```python
from build123d import *

# Parameters (mm, degrees)
ESQUISSE1_R                  = 30.9
ESQUISSE1_R_2                = 12.5
BOSS_EXTRU_1_DEPTH           = 0.6
ESQUISSE2_R                  = 2.1
ENL_V_MAT_EXTRU_1_DEPTH      = 44.703317952
R_P_TITION_CIRCULAIRE1_COUNT = 4


with BuildPart() as part:
    # Esquisse1 → Boss.-Extru.1 (new body)
    with BuildSketch(Plane.XY):
        Circle(ESQUISSE1_R)
        Circle(ESQUISSE1_R_2, mode=Mode.SUBTRACT)
    extrude(amount=BOSS_EXTRU_1_DEPTH)

    # Esquisse2 → Enlèv. mat.-Extru.1 (cut, through all)
    with BuildSketch(Plane.XY.offset(0.6)):
        with Locations((0, 16)):
            Circle(ESQUISSE2_R)
        with Locations((0, 24)):
            Circle(ESQUISSE2_R)
    enl_v_mat_extru_1 = extrude(amount=-ENL_V_MAT_EXTRU_1_DEPTH, mode=Mode.SUBTRACT)

    # Répétition circulaire1: Enlèv. mat.-Extru.1 ×4 about axis
    r_p_tition_circulaire1_axis = Axis((0, 0, 0), (0, 0, 1))
    for i in range(1, R_P_TITION_CIRCULAIRE1_COUNT):
        add(enl_v_mat_extru_1.rotate(r_p_tition_circulaire1_axis, i * 360 / R_P_TITION_CIRCULAIRE1_COUNT), mode=Mode.SUBTRACT)


solid = part.part
```
Model file for the job. Use its own axes, mm. Round coordinates to 2 decimals unless told otherwise and drop trailing zeros. Loops run counter-clockwise (first coordinate to the right, second up) from the corner with the lowest first, then second, coordinate; pieces in that order, holes last. Notation, with made-up numbers: M -4.75,24 L 36.25,24 A18 ccw 36.25,43 Z; hole C -37,-18.5 d8. An arc over 180 degrees is marked long. Put each result on its own line as item: value. Start each with the question number.
Item 1: Drill centre lines: line 1 along Y through (x, z) = (0, 0.2); line 2 along X through (y, z) = (-3.5, 0.45); line 3 along Y through (x, z) = (-9.5, 0.3). Where is each one in solid material? Low to high.
Item 2: Cut at A-A (x = 0). List the corners of the cut face in (y, z).
Item 3: Mould opens along Y. For faces 1 (the face through (-1.13, -25.77, 0.3)), 2 (the face through (-24.521, -18.802, 0.296)), 3 (the face through (0, -13, 0.6)) say: released by +Y, released by -Y, zero draft, split by the parting line, or undercut.
Item 4: Cut at C-C (y = 24). List the corners of the cut face in (x, z).
Item 5: Drop a flat-ended pin along its axis: P1, Ø4, axis at x = 16, y = 0, coming from the +Z side. Give the stop position or say it passes through.
Item 6: Cut at B-B (z = 0.4). Give the number of separate pieces and of enclosed holes in the cut face, then the cut area to 3 significant figures.
Answer block:
1. line 1: -30.9 to -26.1, -21.9 to -18.1, -13.9 to -12.5, 12.5 to 13.9, 18.1 to 21.9, 26.1 to 30.9
1. line 2: -30.7 to -12, 12 to 30.7
1. line 3: -29.4 to -8.12, 8.12 to 29.4
2. outline: M -30.9,0 L -26.1,0 L -26.1,0.6 L -30.9,0.6 Z; M -21.9,0 L -18.1,0 L -18.1,0.6 L -21.9,0.6 Z; M -13.9,0 L -12.5,0 L -12.5,0.6 L -13.9,0.6 Z; M 12.5,0 L 13.9,0 L 13.9,0.6 L 12.5,0.6 Z; M 18.1,0 L 21.9,0 L 21.9,0.6 L 18.1,0.6 Z; M 26.1,0 L 30.9,0 L 30.9,0.6 L 26.1,0.6 Z
3. face 1: undercut
3. face 2: split by the parting line
3. face 3: zero draft
4. outline: M -19.46,0 L -2.1,0 L -2.1,0.6 L -19.46,0.6 Z; M 2.1,0 L 19.46,0 L 19.46,0.6 L 2.1,0.6 Z
5. P1: through
6. separate pieces: 1
6. enclosed holes: 9
6. area: 2,400 mm2
